Input: part model. Units: mm. Frame: model coordinates. Face numbers are marked on the shaded views. Give positions to 0.01 mm unless a question says otherwise; leave off trailing zeros. Loops run counter-clockwise (first coordinate to the right, second up) from the corner with the lowest first, then second, coordinate; pieces in that order, holes last. Notation, with made-up numbers: (47, 39) -> (58, 39) arc R16 cw to (58, 64) -> close; hole circle Ø3 at (8.5, -2.75). An arc over 180 degrees is marked (long way). Answer as a JSON object with one key per item and string values.
```python
from build123d import *

# Parameters (mm, degrees)
SKETCH2_W           = 68
SKETCH2_H           = 16
BOSS_EXTRUDE1_DEPTH = 2
SKETCH3_W           = 68
SKETCH3_H           = 16
SKETCH3_W_2         = 60.2
SKETCH3_H_2         = 8.2
BOSS_EXTRUDE2_DEPTH = 3
SKETCH4_R           = 0.9
CUT_EXTRUDE1_DEPTH  = 36.057096286
SKETCH5_W           = 21.74313044
SKETCH5_H           = 18
BOSS_EXTRUDE3_DEPTH = 5
SKETCH6_W           = 13
SKETCH6_H           = 5
CUT_EXTRUDE3_DEPTH  = 21.743130441
SKETCH7_W           = 1.5
SKETCH7_H           = 1
BOSS_EXTRUDE4_DEPTH = 21.743130441
CHAMFER1_SIZE       = 3
SKETCH8_W           = 3.9
SKETCH8_H           = 8.2
CUT_EXTRUDE4_DEPTH  = 3
FILLET1_R           = 2
CHAMFER2_SIZE       = 1


with BuildPart() as part:
    # Sketch2 → Boss-Extrude1 (new body)
    with BuildSketch(Plane(origin=(0, 0, 0), x_dir=(1, 0, 0), z_dir=(0, 1, 0))):
        Rectangle(SKETCH2_W, SKETCH2_H)
    extrude(amount=BOSS_EXTRUDE1_DEPTH)

    # Sketch3 → Boss-Extrude2 (add)
    with BuildSketch(Plane(origin=(0, 2, 0), x_dir=(1, 0, 0), z_dir=(0, 1, 0))):
        Rectangle(SKETCH3_W, SKETCH3_H)
        Rectangle(SKETCH3_W_2, SKETCH3_H_2, mode=Mode.SUBTRACT)
    extrude(amount=BOSS_EXTRUDE2_DEPTH)

    # Sketch4 → Cut-Extrude1 (cut, through all)
    with BuildSketch(Plane(origin=(0, 2, 0), x_dir=(1, 0, 0), z_dir=(0, 1, 0))):
        with Locations(Location((-24.8, -2.2, 0), (0, 0, 270))):
            Circle(SKETCH4_R)
        with Locations(Location((22.8, 2.2, 0), (0, 0, 270))):
            Circle(SKETCH4_R)
    extrude(amount=-CUT_EXTRUDE1_DEPTH, mode=Mode.SUBTRACT)

    # Sketch5 → Boss-Extrude3 (add)
    with BuildSketch(Plane.XZ):
        Rectangle(SKETCH5_W, SKETCH5_H)
    extrude(amount=BOSS_EXTRUDE3_DEPTH)

    # Sketch6 → Cut-Extrude3 (cut)
    with BuildSketch(Plane.ZY.offset(10.87156522)):
        with Locations((0, -2.5)):
            Rectangle(SKETCH6_W, SKETCH6_H)
    extrude(amount=-CUT_EXTRUDE3_DEPTH, mode=Mode.SUBTRACT)

    # Sketch7 → Boss-Extrude4 (add)
    with BuildSketch(Plane.ZY.offset(10.87156522)):
        with Locations((-5.75, -2.5)):
            Rectangle(SKETCH7_W, SKETCH7_H)
        with Locations((5.75, -2.5)):
            Rectangle(SKETCH7_W, SKETCH7_H)
    extrude(amount=-BOSS_EXTRUDE4_DEPTH)

    # Chamfer1
    # the kernel refuses this chamfer: 3 mm, written as the material it adds along each edge
    with BuildSketch(Plane(origin=(10.87156522, 0, 8), x_dir=(0, 0.9996219169112968, -0.02749587661058649), z_dir=(-1, 0, 0))) as chamfer1_piece_1_section:
        Polygon((CHAMFER1_SIZE * 0.999621916911, -CHAMFER1_SIZE * 0.0274958766106), (-CHAMFER1_SIZE * 0.0274958766106, -CHAMFER1_SIZE * 0.999621916911), (0, 0), align=None)
    chamfer1_piece_1 = extrude(amount=21.743130441, mode=Mode.PRIVATE)
    chamfer1_piece_1 = split(chamfer1_piece_1, bisect_by=Plane(origin=(0, 1.266666667, 9), z_dir=(0, 0, -1)), keep=Keep.TOP, mode=Mode.PRIVATE)
    add(chamfer1_piece_1)
    with BuildSketch(Plane(origin=(-10.87156522, 0, -8), x_dir=(0, 0.9996219169112968, 0.02749587661058649), z_dir=(1, 0, 0))) as chamfer1_piece_2_section:
        Polygon((CHAMFER1_SIZE * 0.999621916911, -CHAMFER1_SIZE * 0.0274958766106), (-CHAMFER1_SIZE * 0.0274958766106, -CHAMFER1_SIZE * 0.999621916911), (0, 0), align=None)
    chamfer1_piece_2 = extrude(amount=21.743130441, mode=Mode.PRIVATE)
    chamfer1_piece_2 = split(chamfer1_piece_2, bisect_by=Plane(origin=(0, 1.266666667, -9), z_dir=(0, 0, 1)), keep=Keep.TOP, mode=Mode.PRIVATE)
    add(chamfer1_piece_2)

    # Sketch8 → Cut-Extrude4 (cut)
    with BuildSketch(Plane(origin=(0, 5, 0), x_dir=(1, 0, 0), z_dir=(0, 1, 0))):
        with Locations((32.05, 0)):
            Rectangle(SKETCH8_W, SKETCH8_H)
    extrude(amount=-CUT_EXTRUDE4_DEPTH, mode=Mode.SUBTRACT)

    # Fillet1
    fillet1_edges = [part.edges().sort_by_distance(p)[0] for p in [
        (34, 2.5, 8),
        (-34, 2.5, 8),
        (-34, 2.5, -8),
        (34, 2.5, -8),
    ]]
    fillet(fillet1_edges, radius=FILLET1_R)

    # Chamfer2
    chamfer2_edges = [part.edges().sort_by_distance(p)[0] for p in [
        (34, 5, -5.05),
        (34, 5, 5.05),
        (0, 5, 8),
        (0, 5, -8),
        (-34, 5, 0),
        (-33.414213562, 5, 7.414213562),
        (-33.414213562, 5, -7.414213562),
        (33.414213562, 5, -7.414213562),
        (33.414213562, 5, 7.414213562),
    ]]
    chamfer(chamfer2_edges, length=CHAMFER2_SIZE)


solid = part.part
```
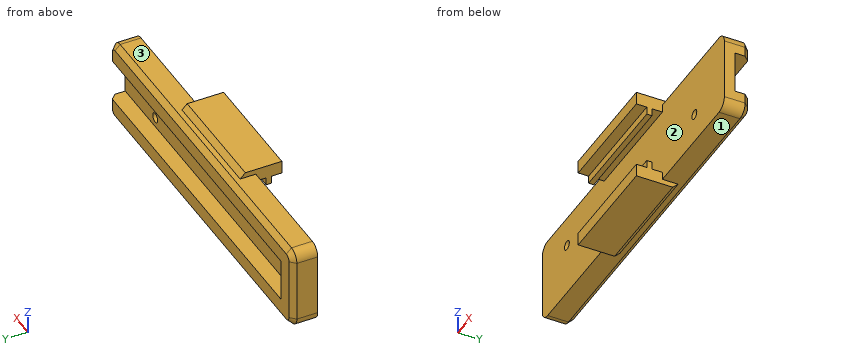
Q1. Draft query along Z for the marked faces 1, 2 and 3. Return one class per face: +Z half, -Z half, draft (parallel to the pull), parting line (faces both ways), or undercut.
Evaluation:
{"face 1": "-Z half", "face 2": "undercut", "face 3": "+Z half"}
Q2. Section C-C, the plane y = -0.75. Return the cut outline in (x, z).
Evaluation:
{"outline": "(-10.87, -9) -> (10.87, -9) -> (10.87, -6.5) -> (-10.87, -6.5) -> close; (-10.87, 6.5) -> (10.87, 6.5) -> (10.87, 9) -> (-10.87, 9) -> close"}
Q3. Section B-B, the plane x = 22.8. Return the cut outline in (y, z), then the cut area to 3 significant figures.
Evaluation:
{"outline": "(0, -8) -> (4, -8) -> (5, -7) -> (5, -4.1) -> (2, -4.1) -> (2, -3.1) -> (0, -3.1) -> close; (0, -1.3) -> (2, -1.3) -> (2, 4.1) -> (5, 4.1) -> (5, 7) -> (4, 8) -> (0, 8) -> close", "area": "50.8 mm2"}
Q4. Section A-A, the plane z = 2.2. Return the cut outline in (x, y), then the cut area to 3 significant figures.
Evaluation:
{"outline": "(-34, 0) -> (-25.7, 0) -> (-25.7, 2) -> (-30.1, 2) -> (-30.1, 5) -> (-33, 5) -> (-34, 4) -> close; (-23.9, 0) -> (34, 0) -> (34, 2) -> (-23.9, 2) -> close", "area": "144 mm2"}
Q5. Pin query (flat end, axial travel): pin 1 (2 mm diameter, centred on y = -2.5, z = 6.5, fed in from +X); pin 2 (5 mm diameter, centred on x = -7.5, z = -1.5, fed in from -Y); pin 3 (6 mm diameter, centred on x = -22, y = -1.5, fed in from -Z); pin 4 (1.4 mm diameter, centred on x = 22.8, z = -2.2, fed in from +Y). Return the tip coordinate at first contact, or that it passes through.
Evaluation:
{"pin 1": "stops at x = 10.87", "pin 2": "stops at y = 0", "pin 3": "stops at z = -8", "pin 4": "passes through"}
Q6. Ray query, line 1 along Z through (x, y) = (14.5, 4); line 2 along X through (y, z) = (0.7, 2.2); line 3 along X through (y, z) = (1.1, -2.2). Return the intervals inside material, ascending.
Evaluation:
{"line 1": "z = -8 to -4.1, 4.1 to 8", "line 2": "x = -34 to -25.7, -23.9 to 34", "line 3": "x = -34 to 21.9, 23.7 to 34"}
Q7. Section D-D, the plane x = -28.5. Return the cut outline in (y, z), then the cut area to 3 significant figures.
Evaluation:
{"outline": "(0, -8) -> (4, -8) -> (5, -7) -> (5, -4.1) -> (2, -4.1) -> (2, 4.1) -> (5, 4.1) -> (5, 7) -> (4, 8) -> (0, 8) -> close", "area": "54.4 mm2"}
